```python
from build123d import *

# Parameters (mm, degrees)
PAD_DEPTH = 2200


with BuildPart() as part:
    # Sketch → Pad (new body)
    with BuildSketch(Plane.XZ):
        with BuildLine():
            ThreePointArc((5.001278, -8.659516), (-0.001476, 10), (-4.998722, -8.660992))
            Line((-4.998722, -8.660992), (-12.7, -22))
            Line((-22.5, -22), (-12.7, -22))
            Line((-22.5, -27), (-22.5, -22))
            Line((-22.5, -27), (22.5, -27))
            Line((22.5, -27), (22.5, -22))
            Line((12.703402, -22), (22.5, -22))
            Line((5.001278, -8.659516), (12.703402, -22))
        make_face()
    extrude(amount=PAD_DEPTH)


solid = part.part
```
Source: CAD feature listing. Evaluate the final solid. Frame: model axes, mm. Give positions to 0.01 mm unless a question says otherwise; leave off trailing zeros. Loops run counter-clockwise (first coordinate to the right, second up) from the corner with the lowest first, then second, coordinate; pieces in that order, holes last. Notation, with made-up numbers: (79, 63) -> (122, 63) arc R10 ccw to (122, 82) -> close; hole circle Ø6 at (78, -33). An arc over 180 degrees is marked (long way). Use a Markdown table: item, result. Add a question column.
(1) First-contact query: pin 1 Ø5 at (x, y) = (-18, -924.5) entering from +Z; pin 2 Ø6 at (y, z) = (-340.5, 1.5) entering from +X; pin 3 Ø1 at (y, z) = (-1564.5, -9.5) entering from +X; pin 4 Ø5 at (x, z) = (14, -16.5) entering from +Y. Flat tips, straight axial feed; report the tip coordinate or a pass-through.
(2) Ray query, line 1 (Z direction, x = -15, y = -559); line 2 (X direction, y = -140, z = -21.5); line 3 (Z direction, x = -7.5, y = -800.5). Return the intervals inside material, ascending.
(3) Section query B-B (z = 0). Output: boundary loops of the cut face in (x, y), then the cut area to 3 significant figures.
(4) Section query A-A (y = -1789). Output: boundary loops of the cut face in (x, z).
Checked values:
| question | item | result |
|---|---|---|
| 1 | pin 1 | z = -22 |
| 1 | pin 2 | x = 10 |
| 1 | pin 3 | x = 5.78 |
| 1 | pin 4 | through |
| 2 | line 1 | -27 to -22 |
| 2 | line 2 | -12.41 to 12.41 |
| 2 | line 3 | -27 to -12.99, -6.61 to 6.61 |
| 3 | outline | (-10, -2200) -> (10, -2200) -> (10, 0) -> (-10, 0) -> close |
| 3 | area | 44,000 mm^2 |
| 4 | outline | (-22.5, -27) -> (22.5, -27) -> (22.5, -22) -> (12.7, -22) -> (5, -8.66) arc R10 ccw (long way) to (-5, -8.66) -> (-12.7, -22) -> (-22.5, -22) -> close |
